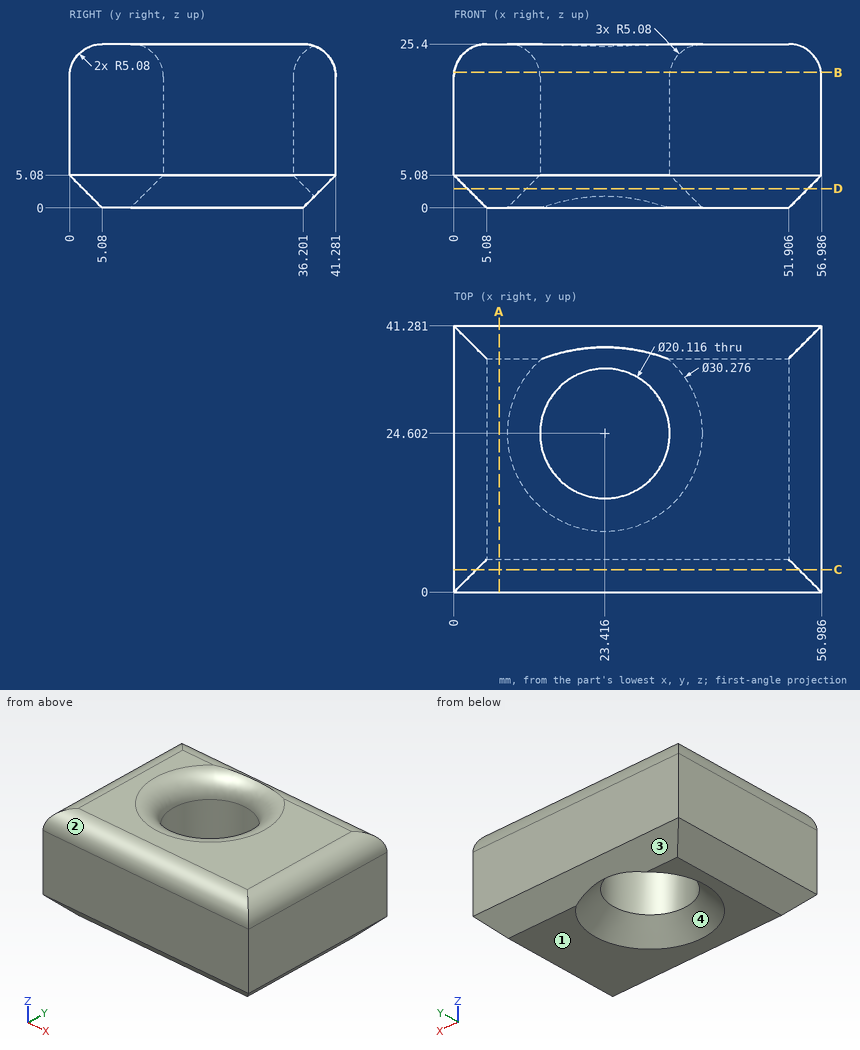
For this review, use the dimensioned drawing (mm, ordinates from the lowest corner) and the shaded views. Give positions to 0.01 mm unless a question says otherwise; leave off trailing zeros. Order: outer loops, then holes, each group sorted by start corner. A loop starts at its lowest first (then second) coordinate and runs counter-clockwise, first axis right, second up. Notation, with made-up numbers: (-1.5, 73) - (54.5, 73) arc R9 cw to (54.5, 77) - close; hole circle Ø6 at (73.25, 21). An arc over 180 degrees is marked (long way). Use CSV: the item, a comma, the result in double quotes. Start each with the question number.
Q1. For P1, Ø3, axis at x = 34.5, y = 24, coming from the -Z side, flat-tipped, find the tip position at first contact; note if it passes through.
Q2. Draft analysis for pull direction Y (two halves, no side actions). For the marked faces 1, 2, 3 and 4, state which applies: pulls with the +Y half, pulls with the -Y half, needs draft (parallel to the pull), parting line crosses it, or undercut.
Q3. For line 1 (X direction, y = 21.5, z = 6.75) (1 decimal); line 2 (X direction, y = 32.5, z = 19) (1 decimal); line 3 (Y direction, x = 26, z = 13), list the stretches that pass through material, from the lowest coordinate up.
Q4. Take a section at B-B (z = 21). State the section outline as (x, y) points (1 decimal).
Q5. Take a section at A-A (x = 7). State the section outline as (y, z) points, and give its area (3 significant figures).
Q6. Take a section at C-C (y = 3.5). State the section outline as (x, z) points (1 decimal), and give its area (3 significant figures).
Q7. Take a section at D-D (z = 3). State the section outline as (x, y) points (1 decimal).
Calculated:
1,P1,"stops at z = 2.54"
2,face 1,"needs draft"
2,face 2,"pulls with the -Y half"
2,face 3,"pulls with the +Y half"
2,face 4,"undercut"
3,line 1,"x = 0 to 13.8, 33 to 57"
3,line 2,"x = 0 to 17.2, 29.6 to 57"
3,line 3,"y = 0 to 14.88, 34.32 to 41.28"
4,outline,"(0, 0) - (56.9, 0) - (56.9, 41.2) - (0, 41.2) - close; hole circle Ø20.2 at (23.4, 24.6)"
5,outline,"(0, 5.08) - (5.08, 0) - (36.2, 0) - (41.28, 5.08) - (41.28, 20.32) arc R5.08 ccw to (36.2, 25.4) - (5.08, 25.4) arc R5.08 ccw to (0, 20.32) - close"
5,area,"1,010 mm²"
6,outline,"(0, 5.1) - (3.5, 1.6) - (53.5, 1.6) - (57, 5.1) - (57, 20.3) arc R5.1 ccw to (53.5, 25.1) - (3.5, 25.1) arc R5.1 ccw to (0, 20.3) - close"
6,area,"1,320 mm²"
7,outline,"(2.1, 2.1) - (54.9, 2.1) - (54.9, 39.2) - (2.1, 39.2) - close; hole circle Ø24.3 at (23.4, 24.6)"
